```python
from build123d import *

# Parameters (mm, degrees)
EXTRUDE_1_DEPTH      = 9
EXTRUDE_1_DEPTH_BACK = 9
SKETCH_6_R           = 2.25
CUT_EXTRUDE_1_DEPTH  = 44.370496884
SKETCH_7_W           = 20
SKETCH_7_H           = 12
CUT_EXTRUDE_2_DEPTH  = 23
SKETCH_8_W           = 6
SKETCH_8_H           = 14
EXTRUDE_2_DEPTH      = 3
FILLET_1_R           = 2


with BuildPart() as part:
    # Sketch 3 → Extrude 1 (new, two sides: drawn at the far end of the back side and taken through both)
    with BuildSketch(Plane.XY.offset(-EXTRUDE_1_DEPTH_BACK)):
        Polygon((0, 0), (30, 0), (30, 3), (3, 30), (0, 30), align=None)
    extrude(amount=EXTRUDE_1_DEPTH + EXTRUDE_1_DEPTH_BACK)

    # Sketch 6 → Cut-Extrude 1 (cut, through all)
    with BuildSketch(Plane.ZY):
        with Locations(Location((0, 20, 0), (0, 0, 270))):
            Circle(SKETCH_6_R)
    cut_extrude_1 = extrude(amount=-CUT_EXTRUDE_1_DEPTH, mode=Mode.SUBTRACT)

    # Sketch 7 → Cut-Extrude 2 (cut)
    with BuildSketch(Plane(origin=(0, 30, 0), x_dir=(1, 0, 0), z_dir=(0, 1, 0))):
        with Locations((17, 0)):
            Rectangle(SKETCH_7_W, SKETCH_7_H)
    extrude(amount=-CUT_EXTRUDE_2_DEPTH, mode=Mode.SUBTRACT)

    # Sketch 8 → Extrude 2 (add)
    with BuildSketch(Plane.ZY):
        with Locations((0, 7)):
            Rectangle(SKETCH_8_W, SKETCH_8_H)
    extrude_2 = extrude(amount=EXTRUDE_2_DEPTH)

    # Mirror 1: Cut-Extrude 1, Extrude 2 across plane
    add(cut_extrude_1.mirror(Plane(origin=(0, 0, 0), x_dir=(0, 0, 1), z_dir=(0.7071067811865476, -0.7071067811865475, 0))), mode=Mode.SUBTRACT)
    add(extrude_2.mirror(Plane(origin=(0, 0, 0), x_dir=(0, 0, 1), z_dir=(0.7071067811865476, -0.7071067811865475, 0))))

    # Fillet 1
    fillet_1_edges = [part.edges().sort_by_distance(p)[0] for p in [
        (3, 30, 0),
        (30, 3, 0),
    ]]
    fillet(fillet_1_edges, radius=FILLET_1_R)


solid = part.part
```
Part model, mm, in its own coordinate system. A direction names the side the tool comes from. Round coordinates to 2 decimals unless told otherwise and drop trailing zeros. Write each loop counter-clockwise with the first axis right and the second up, starting at its lowest first coordinate (ties: lowest second). Pieces come first, ordered by that corner, then holes. Notation, with made-up numbers: (-5.75, -11.5) -> (51.25, -11.5) arc R10 ccw to (51.25, 5.5) -> close; hole circle Ø6 at (12.25, -34). An arc over 180 degrees is marked (long way). Return JSON: item names as keys, results as strings. Group by question number.
Q1. Saw through at D-D on y = 4. Write the cut outline in (x, z).
Q2. Mould opens along Y. For faces 1 (the flat face through (14, -1, 0)), 2 (the flat face through (7, -3, 0)), 3 (the cylindrical face through (3.451, 17.854, 0.676)), 4 (the flat face through (17, 16, -8)) say: pulls with the +Y half, pulls with the -Y half, needs draft (parallel to the pull), parting line crosses it, or undercut.
Q3. Saw through at B-B on z = 0. Write the cut outline in (x, y).
Q4. Which spindle directions (+Z, -Z, +X, -X, +Y, -Y) get a long thin tool onto all of the face, cutting with end or side? Do faces 5 (the flat face through (16, 7, 0)), 6 (the flat face through (-2, 0, 0)), 7 (the flat face through (7, -1, 3)), 8 (the flat face through (-1, 14, 0)). Say none if no direction does.
Q5. Pin check, flat tips, straight feed: pin 1 (2.5 mm diameter, centred on x = 5, y = -1.5, fed in from -Z); pin 2 (1.5 mm diameter, centred on x = -1.5, z = -1, fed in from -Y); pin 3 (3.5 mm diameter, centred on x = 16, z = -2, fed in from +Y). Stop position of each tip, or through.
Q6. Probe L1, parallel to Z at x = 20, y = 5; L2, parallel to Y at x = 18, z = -3.5. List the from-to ranges inside material, lowest first. Write a range as [from, to].
Q7. Saw through at A-A on y = 20. Write the cut outline in (x, z), plus the area to 4 significant figures.
Answer:
{
 "1": {"outline": "(-3, -3) -> (0, -3) -> (0, -9) -> (29, -9) -> (29, 9) -> (0, 9) -> (0, 3) -> (-3, 3) -> close; hole circle Ø4.5 at (20, 0)"},
 "2": {"face 1": "needs draft", "face 2": "pulls with the -Y half", "face 3": "undercut", "face 4": "pulls with the +Y half"},
 "3": {"outline": "(-3, 0) -> (0, 0) -> (0, -3) -> (14, -3) -> (14, 0) -> (17.75, 0) -> (17.75, 7) -> (7, 7) -> (7, 17.75) -> (0, 17.75) -> (0, 14) -> (-3, 14) -> close; (0, 22.25) -> (7, 22.25) -> (7, 26) -> (3.59, 29.41) arc R2 ccw to (2.17, 30) -> (0, 30) -> close; (22.25, 0) -> (30, 0) -> (30, 2.17) arc R2 ccw to (29.41, 3.59) -> (26, 7) -> (22.25, 7) -> close"},
 "4": {"face 5": "+X, +Y", "face 6": "+Z, -Z, -X, -Y", "face 7": "+Z, +X, -X, -Y", "face 8": "+Z, -Z, -X, +Y"},
 "5": {"pin 1": "z = -3", "pin 2": "y = 0", "pin 3": "y = 7"},
 "6": {"L1": "[-9, -2.25], [2.25, 9]", "L2": "[0, 7]"},
 "7": {"outline": "(0, -9) -> (13, -9) -> (13, -6) -> (7, -6) -> (7, -2.25) -> (0, -2.25) -> close; (0, 2.25) -> (7, 2.25) -> (7, 6) -> (13, 6) -> (13, 9) -> (0, 9) -> close", "area": "130.5 mm2"}
}
